Verification items for the finished model (mm, model axes). Give positions to 0.01 mm unless a question says otherwise; leave off trailing zeros. Write each loop counter-clockwise with the first axis right and the second up, starting at its lowest first coordinate (ties: lowest second). Pieces come first, ordered by that corner, then holes.
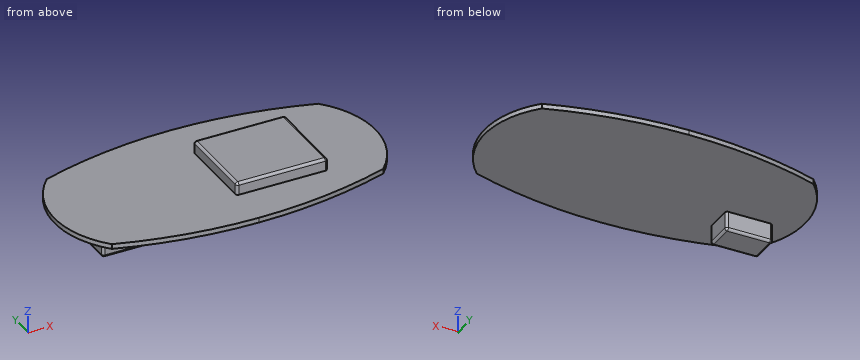
Autodesk Inventor part; units mm, degrees
ref_plane "YZ Plane" through (0, 0, 0) normal (1, 0, 0) x (0, 1, 0)
ref_plane "XZ Plane" through (0, 0, 0) normal (0, 1, 0) x (-1, 0, 0)
ref_plane "XY Plane" through (0, 0, 0) normal (0, 0, 1) x (1, 0, 0)
sketch "Boceto1" plane through (0, 0, 0) normal (0, 0, 1) x (1, 0, 0)
  arc A0 (60, 29.35) -> (32.5, 33.7) centre (32.5, -55.4003) ccw
  arc A1 (32.5, 33.7) -> (5, 29.35) centre (32.5, -55.4003) ccw
  arc A2 (32.5, 0) -> (60, 4.35) centre (32.5, 89.1003) ccw
  arc A3 (60, 4.35) -> (60, 29.35) centre (46.875, 16.85) ccw
  arc A4 (5, 4.35) -> (32.5, 0) centre (32.5, 89.1003) ccw
  arc A5 (5, 29.35) -> (5, 4.35) centre (18.125, 16.85) ccw
  line L0 (32.5, 16.85) -> (32.5, 8.6)
  line L1 (32.5, 8.6) -> (32.5, 25.1)
  line L2 (32.5, 25.1) -> (51, 25.1)
  line L3 (51, 25.1) -> (51, 8.6)
  line L4 (51, 8.6) -> (32.5, 8.6)
  line L5 (32.5, 8.6) -> (32.5, 25.1)
  point P0 (0, 0)
  dimension "d6" = 8.25
  dimension "d7" = 16.5
extrude "Extrusión1" add sketch "Boceto1" along normal blind 2.5 and the other way blind 1 contours L1 L2 L3 L4 L0
extrude "Extrusión2" add sketch "Boceto1" against normal blind 1
sketch "Boceto2" plane through (0, 0, -1) normal (0, 0, -1) x (-1, 0, 0)
  arc A0 (-5, 4.35) -> (-5, 29.35) centre (-18.125, 16.85) ccw
  line L0 (0, 16.85) -> (-5, 16.85)
  line L1 (-5, 16.85) -> (-5, 13.85)
  line L2 (-5, 13.85) -> (-14.5, 13.85)
  line L3 (-14.5, 13.85) -> (-14.5, 7.85)
  line L4 (-14.5, 7.85) -> (-5, 7.85)
  line L5 (-5, 7.85) -> (-5, 13.85)
  line L6 (-5, 13.85) -> (-14.5, 13.85)
  line L7 (-14.5, 13.85) -> (-14.5, 7.85)
  point P0 (0, 0)
  dimension "d14" = 5
  dimension "d15" = 3
  dimension "d16" = 9.5
  dimension "d18" = 6
extrude "Extrusión3" add sketch "Boceto2" along normal blind 3.8
fillet "Empalme1" radius 0.5 16 edges at (5, 13.85, -2.9) (14.5, 13.85, -2.9) (9.75, 13.85, -4.8) (9.75, 7.85, -4.8) (14.5, 10.85, -4.8) (5, 10.85, -4.8) (41.75, 25.1, 2.5) (51, 16.85, 2.5) (41.75, 8.6, 2.5) (32.5, 16.85, 2.5) (32.5, 25.1, 1.25) (51, 25.1, 1.25) (32.5, 8.6, 1.25) (51, 8.6, 1.25) (5, 7.85, -2.9) (14.5, 7.85, -2.9)
properties part number "Bluetooth"
Item 1: Depth check by flat-ended pin: pin 1 (0.6 mm diameter, centred on y = 13, z = 1, fed in from +X); pin 2 (4 mm diameter, centred on y = 19.5, z = -1.5, fed in from +X); pin 3 (2 mm diameter, centred on x = 27.5, y = 22.5, fed in from +Z). Enter the tip coordinate at first touch or a pass-through.
Answer key:
pin 1: stops at x = 51
pin 2: stops at x = 64.99
pin 3: stops at z = 0
Item 2: Sectioned sample at D-D on z = 1. Record the cut outline in (x, y), then the cut area to 3 significant figures.
Answer key:
outline: (32.5, 9.1) arc R0.5 ccw to (33, 8.6) - (50.5, 8.6) arc R0.5 ccw to (51, 9.1) - (51, 24.6) arc R0.5 ccw to (50.5, 25.1) - (33, 25.1) arc R0.5 ccw to (32.5, 24.6) - close
area: 305 mm2
Item 3: Sectioned sample at A-A on z = -2.5. Record the cut outline in (x, y), then the cut area to 3 significant figures.
Answer key:
outline: (5, 8.35) arc R0.5 ccw to (5.5, 7.85) - (14, 7.85) arc R0.5 ccw to (14.5, 8.35) - (14.5, 13.35) arc R0.5 ccw to (14, 13.85) - (5.5, 13.85) arc R0.5 ccw to (5, 13.35) - close
area: 56.8 mm2
Item 4: Sectioned sample at C-C on x = 44. Record the cut outline in (y, z).
Answer key:
outline: (0.75, -1) - (32.95, -1) - (32.95, 0) - (25.1, 0) - (25.1, 2) arc R0.5 ccw to (24.6, 2.5) - (9.1, 2.5) arc R0.5 ccw to (8.6, 2) - (8.6, 0) - (0.75, 0) - close
Item 5: Scan lines: line 1 along Y through (x, z) = (10, -1.5); line 2 along Y through (x, z) = (5, -0.5); line 3 along Z through (x, y) = (16, 8.5). Record each from-to range of solid material in increasing order.
Answer key:
line 1: y = 7.85 to 13.85
line 2: y = 4.35 to 29.35
line 3: z = -1 to 0
Item 6: Sectioned sample at B-B on y = 18.5. Record the cut outline in (x, z), then the cut area to 3 significant figures.
Answer key:
outline: (0.08, -1) - (64.92, -1) - (64.92, 0) - (51, 0) - (51, 2) arc R0.5 ccw to (50.5, 2.5) - (33, 2.5) arc R0.5 ccw to (32.5, 2) - (32.5, 0) - (0.08, 0) - close
area: 111 mm2
